Autodesk Inventor part; units mm, degrees
ref_plane "YZ Plane" through (0, 0, 0) normal (1, 0, 0) x (0, 1, 0)
ref_plane "XZ Plane" through (0, 0, 0) normal (0, 1, 0) x (-1, 0, 0)
ref_plane "XY Plane" through (0, 0, 0) normal (0, 0, 1) x (1, 0, 0)
sketch "Sketch1" plane through (0, 0, 0) normal (0, 1, 0) x (-1, 0, 0)
  line L0 (0, 0) -> (-25.4, 0)
  line L1 (-25.4, -35.921) -> (-25.4, -127)
  line L2 (-25.4, -152.4) -> (0, -152.4)
  line L3 (0, -152.4) -> (0, 0)
  line L4 (0, -152.4) -> (-152.4, -152.4)
  line L5 (-152.4, -152.4) -> (-152.4, -127)
  line L6 (-116.479, -127) -> (-25.4, -127)
  line L7 (0, -127) -> (0, -152.4)
  line L8 (-152.4, -127) -> (-25.4, 0)
  line L9 (-25.4, -35.921) -> (-116.479, -127)
  dimension "d0" = 25.4
  dimension "d1" = 152.4
  dimension "d2" = 152.4
  dimension "d3" = 25.4
  dimension "d4" = 25.4
extrude "Extrusion1" add sketch "Sketch1" along normal blind 1.5875
sketch "Sketch2" plane through (0, 1.5875, 0) normal (0, 1, 0) x (1, 0, 0)
  line L0 (152.4, 152.4) -> (0, 152.4)
  line L1 (0, 152.4) -> (25.4, 152.4)
  line L2 (25.4, 35.921) -> (25.4, 127)
  line L3 (25.4, 152.4) -> (25.4, 127)
  line L4 (25.4, 127) -> (0, 152.4)
  line L5 (25.4, 152.4) -> (0, 127)
  line L6 (0, 152.4) -> (0, 0)
  line L7 (12.7, 139.7) -> (38.1, 139.7)
  line L8 (38.1, 139.7) -> (63.5, 139.7)
  line L9 (63.5, 139.7) -> (88.9, 139.7)
  line L10 (88.9, 139.7) -> (114.3, 139.7)
  line L11 (114.3, 139.7) -> (139.7, 139.7)
  line L12 (12.7, 139.7) -> (12.7, 114.3)
  line L13 (12.7, 114.3) -> (12.7, 88.9)
  line L14 (12.7, 88.9) -> (12.7, 63.5)
  line L15 (12.7, 63.5) -> (12.7, 38.1)
  line L16 (12.7, 38.1) -> (12.7, 12.7)
  circle A0 centre (12.7, 139.7) radius 2.54
  circle A1 centre (38.1, 139.7) radius 2.54
  circle A2 centre (63.5, 139.7) radius 2.54
  circle A3 centre (88.9, 139.7) radius 2.54
  circle A4 centre (114.3, 139.7) radius 2.54
  circle A5 centre (139.7, 139.7) radius 2.54
  circle A6 centre (12.7, 114.3) radius 2.54
  circle A7 centre (12.7, 88.9) radius 2.54
  circle A8 centre (12.7, 63.5) radius 2.54
  circle A9 centre (12.7, 38.1) radius 2.54
  circle A10 centre (12.7, 12.7) radius 2.54
  dimension "d7" = 25.4
  dimension "d8" = 25.4
  dimension "d9" = 25.4
  dimension "d10" = 25.4
  dimension "d11" = 25.4
  dimension "d12" = 25.4
  dimension "d13" = 25.4
  dimension "d14" = 25.4
  dimension "d15" = 25.4
  dimension "d16" = 25.4
  dimension "d17" = 5.08
  dimension "d18" = 5.08
  dimension "d19" = 5.08
  dimension "d20" = 5.08
  dimension "d21" = 5.08
  dimension "d22" = 5.08
  dimension "d23" = 5.08
  dimension "d24" = 5.08
hole "Hole1" at (12.7, 1.5875, -139.7) at (38.1, 1.5875, -139.7) at (63.5, 1.5875, -139.7) at (88.9, 1.5875, -139.7) at (114.3, 1.5875, -139.7) at (12.7, 1.5875, -114.3) at (12.7, 1.5875, -88.9) at (12.7, 1.5875, -63.5) at (12.7, 1.5875, -38.1) direction (0, -1, 0) diameter 5.08 end through all
sketch "Sketch3" plane through (0, 1.5875, 0) normal (0, 1, 0) x (1, 0, 0)
  line L0 (116.479, 127) -> (25.4, 127)
  line L1 (116.479, 127) -> (129.179, 127)
  line L2 (129.179, 127) -> (129.179, 152.4)
  line L3 (152.4, 152.4) -> (0, 152.4)
  line L4 (25.4, 35.921) -> (25.4, 127)
  line L5 (25.4, 35.921) -> (25.4, 23.221)
  line L6 (25.4, 23.221) -> (0, 23.221)
  line L7 (0, 23.221) -> (0, 0)
  line L8 (25.4, 0) -> (152.4, 127)
  line L9 (0, 0) -> (25.4, 0)
  line L10 (25.4, 0) -> (152.4, 127)
  line L11 (152.4, 127) -> (152.4, 152.4)
  line L12 (152.4, 127) -> (152.4, 152.4)
  line L13 (152.4, 152.4) -> (129.179, 152.4)
  line L14 (116.479, 127) -> (25.4, 35.921)
  dimension "d32" = 12.7
  dimension "d33" = 12.7
extrude "Extrusion2" cut sketch "Sketch3" against normal blind 1.5875 contours L1 L2 L3 L11 L8 L9 L7 L6 L5 L14
sketch "Sketch4" plane through (0, 1.5875, 0) normal (0, 1, 0) x (1, 0, 0)
  line L0 (129.179, 127) -> (25.4, 127)
  line L1 (129.179, 127) -> (25.4, 23.221)
  line L2 (25.4, 59.142) -> (93.258, 127)
  line L3 (25.4, 127) -> (25.4, 23.221)
  line L4 (25.4, 59.142) -> (25.4, 23.221)
  point P0 (0, 0)
  dimension "d36" = 25.4
extrude "Extrusion3" add sketch "Sketch4" against normal blind 1.5875 contours L1 L3 L2 L0
fillet "Fillet1" radius 3.175 3 edges at (25.4, 0.7937, -127) (93.258, 0.7937, -127) (25.4, 0.7937, -59.142)
properties part number "Gusset 2B"
Read the model definition and answer for the solid it produces. Units are mm, in the model's axes. A direction names the side the tool comes from. Give positions to 0.01 mm unless a question says otherwise; leave off trailing zeros. Loops run counter-clockwise (first coordinate to the right, second up) from the corner with the lowest first, then second, coordinate; pieces in that order, holes last. Notation, with made-up numbers: (9.5, 47) -> (45.5, 47) arc R9 cw to (45.5, 55) -> close; hole circle Ø7 at (31, -20.5). An arc over 180 degrees is marked (long way). Answer as CSV lines item,"result".
Item 1: Consider line 1 (Z direction, x = 12.7, y = 1); line 2 (X direction, y = 0.85, z = -139.7); line 3 (X direction, y = 0.45, z = -114.5). Determine where each line is inside the solid, lowest interval first. Write a range as [from, to].
Returned:
line 1,"z = [-152.4, -142.24], [-137.16, -116.84], [-111.76, -91.44], [-86.36, -66.04], [-60.96, -40.64], [-35.56, -23.22]"
line 2,"x = [0, 10.16], [15.24, 35.56], [40.64, 60.96], [66.04, 86.36], [91.44, 111.76], [116.84, 129.18]"
line 3,"x = [0, 10.17], [15.23, 25.4], [80.76, 116.68]"
Item 2: For faces 1 (the face through (64, 1.588, -89)), 2 (the face through (27.409, 0.783, -63.854)), determine the directions among +Z, -Z, +X, -X, +Y, -Y from which every point of the face is accessible in a straight line to the end or side of a thin tool.
Returned:
face 1,"+Z, -Z, +X, -X, +Y"
face 2,"+Y, -Y"
Item 3: Find section C-C on y = 1.15. State how many separate pieces and enclosed holes the cut face has, plus the area to 3 significant figures.
Returned:
separate pieces,"1"
enclosed holes,"10"
area,"8,840 mm²"
Item 4: Determine the mould class of faces 3 (the face through (64, 0, -89)), 4 (the face through (78.02, 0.8, -75.84)), 5 (the face through (88.5, 0.8, -125.1)) for opening direction X: +X half, -X half, draft (parallel to the pull), parting line (faces both ways), or undercut.
Returned:
face 3,"draft"
face 4,"+X half"
face 5,"undercut"
Item 5: Find section B-B on z = -139.7. Give the vertices of the cut face in (x, y), plus the area to 3 significant figures.
Returned:
outline,"(0, 0) -> (10.16, 0) -> (10.16, 1.59) -> (0, 1.59) -> close; (15.24, 0) -> (35.56, 0) -> (35.56, 1.59) -> (15.24, 1.59) -> close; (40.64, 0) -> (60.96, 0) -> (60.96, 1.59) -> (40.64, 1.59) -> close; (66.04, 0) -> (86.36, 0) -> (86.36, 1.59) -> (66.04, 1.59) -> close; (91.44, 0) -> (111.76, 0) -> (111.76, 1.59) -> (91.44, 1.59) -> close; (116.84, 0) -> (129.18, 0) -> (129.18, 1.59) -> (116.84, 1.59) -> close"
area,"165 mm²"
Item 6: Find section A-A on x = 12.7. Give the vertices of the cut face in (y, z).
Returned:
outline,"(0, -152.4) -> (1.59, -152.4) -> (1.59, -142.24) -> (0, -142.24) -> close; (0, -137.16) -> (1.59, -137.16) -> (1.59, -116.84) -> (0, -116.84) -> close; (0, -111.76) -> (1.59, -111.76) -> (1.59, -91.44) -> (0, -91.44) -> close; (0, -86.36) -> (1.59, -86.36) -> (1.59, -66.04) -> (0, -66.04) -> close; (0, -60.96) -> (1.59, -60.96) -> (1.59, -40.64) -> (0, -40.64) -> close; (0, -35.56) -> (1.59, -35.56) -> (1.59, -23.22) -> (0, -23.22) -> close"
Item 7: Find section D-D on z = -119. Give the vertices of the cut face in (x, y), plus the area to 3 significant figures.
Returned:
outline,"(0, 0) -> (25.4, 0) -> (25.4, 1.59) -> (0, 1.59) -> close; (85.26, 0) -> (121.18, 0) -> (121.18, 1.59) -> (85.26, 1.59) -> close"
area,"97.3 mm²"
